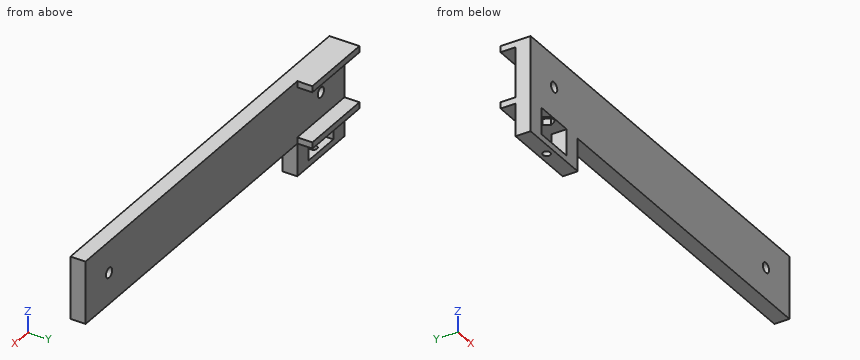
```python
from build123d import *

# Parameters (mm, degrees)
SKETCH1_W           = 30
SKETCH1_H           = 20
SKETCH1_H_2         = 2.5
SKETCH1_W_2         = 7
SKETCH1_H_3         = 10.6
SKETCH1_W_3         = 16
SKETCH1_W_4         = 15
SKETCH1_H_4         = 10
SKETCH1_R           = 2
BOSS_EXTRUDE1_DEPTH = 6
SKETCH1_3_W         = 7
SKETCH1_3_H         = 2.5
SKETCH1_3_W_2       = 30
BOSS_EXTRUDE2_DEPTH = 12
SKETCH3_R           = 1.5
CUT_EXTRUDE2_DEPTH  = 5
CUT_EXTRUDE3_DEPTH  = 2.5
CUT_EXTRUDE1_DEPTH  = 137.99361299


with BuildPart() as part:
    # Sketch1 → Boss-Extrude1 (new body)
    # profile 1 of 13: a face of its own
    with BuildSketch(Plane(origin=(0, 0, 0), x_dir=(1, 0, 0), z_dir=(0, 1, 0))):
        with Locations((-15, -10)):
            Rectangle(SKETCH1_W, SKETCH1_H)
    # profile 2 of 13: a face of its own
    with BuildSketch(Plane(origin=(0, 0, 0), x_dir=(1, 0, 0), z_dir=(0, 1, 0))):
        with Locations((-15, -21.25)):
            Rectangle(SKETCH1_W, SKETCH1_H_2)
    # profile 3 of 13: a face of its own
    with BuildSketch(Plane(origin=(0, 0, 0), x_dir=(1, 0, 0), z_dir=(0, 1, 0))):
        Polygon((-15, 0), (-7, 0), (-7, 2.5), (-23, 2.5), (-23, 0), align=None)
    # profile 4 of 13: a face of its own
    with BuildSketch(Plane(origin=(0, 0, 0), x_dir=(1, 0, 0), z_dir=(0, 1, 0))):
        with Locations((-3.5, 1.25)):
            Rectangle(SKETCH1_W_2, SKETCH1_H_2)
    # profile 5 of 13: a face of its own
    with BuildSketch(Plane(origin=(0, 0, 0), x_dir=(1, 0, 0), z_dir=(0, 1, 0))):
        with Locations((-3.5, 7.8)):
            Rectangle(SKETCH1_W_2, SKETCH1_H_3)
    # profile 6 of 13: a face of its own
    with BuildSketch(Plane(origin=(0, 0, 0), x_dir=(1, 0, 0), z_dir=(0, 1, 0))):
        with Locations((-3.5, 14.35)):
            Rectangle(SKETCH1_W_2, SKETCH1_H_2)
    # profile 7 of 13: a face of its own
    with BuildSketch(Plane(origin=(0, 0, 0), x_dir=(1, 0, 0), z_dir=(0, 1, 0))):
        with Locations((-15, 14.35)):
            Rectangle(SKETCH1_W_3, SKETCH1_H_2)
    # profile 8 of 13: a face of its own
    with BuildSketch(Plane(origin=(0, 0, 0), x_dir=(1, 0, 0), z_dir=(0, 1, 0))):
        with Locations((-26.5, 14.35)):
            Rectangle(SKETCH1_W_2, SKETCH1_H_2)
    # profile 9 of 13: a face of its own
    with BuildSketch(Plane(origin=(0, 0, 0), x_dir=(1, 0, 0), z_dir=(0, 1, 0))):
        with Locations((-26.5, 7.8)):
            Rectangle(SKETCH1_W_2, SKETCH1_H_3)
    # profile 10 of 13: a face of its own
    with BuildSketch(Plane(origin=(0, 0, 0), x_dir=(1, 0, 0), z_dir=(0, 1, 0))):
        with Locations((-26.5, 1.25)):
            Rectangle(SKETCH1_W_2, SKETCH1_H_2)
    # profile 11 of 13: a face of its own
    with BuildSketch(Plane(origin=(0, 0, 0), x_dir=(1, 0, 0), z_dir=(0, 1, 0))):
        with Locations((-22.5, -15)):
            Rectangle(SKETCH1_W_4, SKETCH1_H_4)
    # profile 12 of 13: a face of its own
    with BuildSketch(Plane(origin=(0, 0, 0), x_dir=(1, 0, 0), z_dir=(0, 1, 0))):
        Polygon((-30, -10), (-15, -10), (-15, 0), (-23, 0), (-30, 0), align=None)
    # profile 13 of 13: a face of its own
    with BuildSketch(Plane(origin=(0, 0, 0), x_dir=(1, 0, 0), z_dir=(0, 1, 0))):
        Polygon((135, -22.5), (0, -22.5), (0, -20), (0, 0), (0, 2.5), (135, 2.5), align=None)
        with Locations(Location((120, -10, 0), (0, 0, 270))):
            Circle(SKETCH1_R, mode=Mode.SUBTRACT)
    extrude(amount=BOSS_EXTRUDE1_DEPTH)

    # Sketch1_3 → Boss-Extrude2 (add)
    with BuildSketch(Plane(origin=(0, 0, 0), x_dir=(1, 0, 0), z_dir=(0, 1, 0))):
        with Locations((-3.5, 1.25)):
            Rectangle(SKETCH1_3_W, SKETCH1_3_H)
        Polygon((-15, 0), (-7, 0), (-7, 2.5), (-23, 2.5), (-23, 0), align=None)
        with Locations((-15, -21.25)):
            Rectangle(SKETCH1_3_W_2, SKETCH1_3_H)
        with Locations((-26.5, 1.25)):
            Rectangle(SKETCH1_3_W, SKETCH1_3_H)
    extrude(amount=BOSS_EXTRUDE2_DEPTH)

    # Sketch3 → Cut-Extrude2 (cut)
    with BuildSketch(Plane(origin=(0, 0, -15.6), x_dir=(-1, 0, 0), z_dir=(0, 0, -1))):
        with Locations((15, 3)):
            Circle(SKETCH3_R)
    extrude(amount=-CUT_EXTRUDE2_DEPTH, mode=Mode.SUBTRACT)

    # Sketch4 → Cut-Extrude3 (cut)
    with BuildSketch(Plane(origin=(0, 0, -2.5), x_dir=(-1, 0, 0), z_dir=(0, 0, -1))):
        Polygon((17.886751346, 3), (16.443375673, 5.5), (13.556624327, 5.5), (12.113248654, 3), (13.556624327, 0.5), (16.443375673, 0.5), align=None)
    extrude(amount=-CUT_EXTRUDE3_DEPTH, mode=Mode.SUBTRACT)

    # Sketch2 → Cut-Extrude1 (cut, through all)
    with BuildSketch(Plane(origin=(0, 6, 0), x_dir=(1, 0, 0), z_dir=(0, 1, 0))):
        with BuildLine():
            ThreePointArc((-13, -10), (-15, -8), (-17, -10))
            Line((-17, -10), (-13, -10))
        make_face()
        with BuildLine():
            Line((-13, -10), (-17, -10))
            ThreePointArc((-17, -10), (-15, -12), (-13, -10))
        make_face()
    extrude(amount=-CUT_EXTRUDE1_DEPTH, mode=Mode.SUBTRACT)


solid = part.part
```
CAD build for the part. Positions are in the model's coordinates, mm. Round coordinates to 2 decimals unless told otherwise and drop trailing zeros. Loops run counter-clockwise (first coordinate to the right, second up) from the corner with the lowest first, then second, coordinate; pieces in that order, holes last. Notation, with made-up numbers: M 26.25,-30.5 L 68.25,-30.5 A10 ccw 68.25,-24.5 Z; hole C -18,15.5 d4. An arc over 180 degrees is marked long. Use a Markdown table: item, result. Add a question column.
(1) Cut at D-D (x = 120). Give the cut face in (y, z), and give its area (3 significant figures).
(2) Cut at B-B (z = -8). Give the cut face in (x, y), and give its area (3 significant figures).
(3) Cut at C-C (z = 10). Give the cut face in (x, y), and give its area (3 significant figures).
(4) Flat gauge pins, fed straight in: pin 1 (1 mm diameter, centred on y = 4, z = -11.5, fed in from +X); pin 2 (12.5 mm diameter, centred on x = 28.5, z = 6, fed in from +Y); pin 3 (6 mm diameter, centred on x = 25, y = 7, fed in from -Z); pin 4 (2 mm diameter, centred on x = 49.5, y = 7.5, fed in from +Z). Where does each tip first touch, or does it go through?
(5) Drill centre lines: line 1 (Z direction, x = 0.5, y = 0.5); line 2 (Y direction, x = 63, z = 14); line 3 (X direction, y = 3, z = -7.5). Where is each one in solid material? Low to high.
(6) Cut at A-A (x = -15). Give the cut face in (y, z).
Geometry says:
| question | item | result |
|---|---|---|
| 1 | outline | M 0,-2.5 L 6,-2.5 L 6,8 L 0,8 Z; M 0,12 L 6,12 L 6,22.5 L 0,22.5 Z |
| 1 | area | 126 mm² |
| 2 | outline | M -30,0 L -23,0 L -23,6 L -30,6 Z; M -7,0 L 0,0 L 0,6 L -7,6 Z |
| 2 | area | 84.0 mm² |
| 3 | outline | M -30,0 L -17,0 L -17,6 L -30,6 Z; M -13,0 L 118,0 L 118,6 L -13,6 Z; M 122,0 L 135,0 L 135,6 L 122,6 Z |
| 3 | area | 942 mm² |
| 4 | pin 1 | stops at x = 0 |
| 4 | pin 2 | stops at y = 6 |
| 4 | pin 3 | stops at z = -2.5 |
| 4 | pin 4 | passes through |
| 5 | line 1 | z = -2.5 to 22.5 |
| 5 | line 2 | y = 0 to 6 |
| 5 | line 3 | x = -30 to -23, -7 to 0 |
| 6 | outline | M 0,-15.6 L 1.5,-15.6 L 1.5,-13.1 L 0,-13.1 Z; M 0,-2.5 L 0.5,-2.5 L 0.5,0 L 5.5,0 L 5.5,-2.5 L 12,-2.5 L 12,0 L 6,0 L 6,8 L 0,8 Z; M 0,12 L 6,12 L 6,20 L 12,20 L 12,22.5 L 0,22.5 Z; M 4.5,-15.6 L 6,-15.6 L 6,-13.1 L 4.5,-13.1 Z |
